from build123d import *

# Parameters (mm, degrees)
SKETCH_1_W          = 10
SKETCH_1_H          = 6
EXTRUDE_1_DEPTH     = 11.3
CUT_EXTRUDE_1_REACH = 18.239
SKETCH_3_W          = 3.4
SKETCH_3_H          = 3.4
CUT_EXTRUDE_2_DEPTH = 8
SKETCH_4_R          = 0.5
CUT_EXTRUDE_3_DEPTH = 0.1


with BuildPart() as part:
    # 草图1 → 凸台-拉伸1 (new body)
    with BuildSketch(Plane(origin=(0, 0, 0), x_dir=(1, 0, 0), z_dir=(0, 1, 0))):
        with Locations((5, 3)):
            Rectangle(SKETCH_1_W, SKETCH_1_H)
    extrude(amount=EXTRUDE_1_DEPTH)

    # 草图2 → 切除-拉伸1 (cut, up to next)
    with BuildSketch(Plane(origin=(0, 0, -6), x_dir=(-1, 0, 0), z_dir=(0, 0, -1)), mode=Mode.PRIVATE) as cut_extrude_1_sk1:
        Polygon((-10, 3.8), (-5.669872981, 11.3), (-10, 11.3), align=None)
    cut_extrude_1_tool1 = extrude(cut_extrude_1_sk1.sketch, amount=-CUT_EXTRUDE_1_REACH, mode=Mode.PRIVATE) & part.part
    add(cut_extrude_1_tool1.solids().sort_by_distance((8.556624, 8.8, -6))[0], mode=Mode.SUBTRACT)

    # 草图3 → 切除-拉伸2 (cut)
    with BuildSketch(Plane(origin=(9.145448267, 5.280127019, 0), x_dir=(0, 0, -1), z_dir=(0.8660254037844417, 0.4999999999999948, 0))):
        with Locations((3, 2.621023553)):
            Rectangle(SKETCH_3_W, SKETCH_3_H)
    extrude(amount=-CUT_EXTRUDE_2_DEPTH, mode=Mode.SUBTRACT)

    # 草图4 → 切除-拉伸3 (cut)
    with BuildSketch(Plane.XZ):
        with Locations(Location((5, -3, 0), (0, 0, 270))):
            Circle(SKETCH_4_R)
    extrude(amount=-CUT_EXTRUDE_3_DEPTH, mode=Mode.SUBTRACT)


solid = part.part
Geometry check sheet. Reference: the model listing, model coordinates, mm. A direction names the side the tool comes from. Coordinates: 2 decimals unless noted, no trailing zeros. Order: outer loops, then holes, each group sorted by start corner. A loop starts at its lowest first (then second) coordinate and runs counter-clockwise, first axis right, second up. Notation, with made-up numbers: (85, -39.5) - (118, -39.5) arc R29 ccw to (118, -17.5) - close; hole circle Ø1 at (70, 74). An arc over 180 degrees is marked (long way). One line per item, written item: value.
(1) Thickness scan on probe 1 along X at (y, z) = (0.05, -3); probe 2 along Z at (x, y) = (3.75, 3.75); probe 3 along Y at (x, z) = (6, -2.7). Record the ranges inside material, lowest first. Write a range as from..to.
Data:
probe 1: x = 0..4.5, 5.5..10
probe 2: z = -6..-4.7, -1.3..0
probe 3: y = 0..4.53, 8.45..10.73
(2) Release check for a two-part mould opening along Z. For faces 1 (the face through (4, 6, -6)), 2 (the face through (5.269, 4.106, -2.976)), 3 (the face through (4, 6, 0)), 4 (the face through (3, 11.3, -3)) record: +Z half, -Z half, draft (parallel to the pull), parting line (faces both ways), or undercut.
Data:
face 1: -Z half
face 2: undercut
face 3: +Z half
face 4: draft
(3) Sectioned sample at D-D (y = 7.75). Enter the section's corners in (x, z).
Data:
outline: (0, -6) - (7.72, -6) - (7.72, -4.7) - (4.78, -4.7) - (4.78, -1.3) - (7.72, -1.3) - (7.72, 0) - (0, 0) - close
(4) Access from +Z, -Z, +X, -X, +Y, -Y to the whole of each face (thin tool, end or side, straight path). Record for faces 5 (the face through (8.83, 5.83, -3.04)), 6 (the face through (5, 0.1, -3)), 7 (the face through (0.895, 3.571, -2.976)).
Data:
face 5: +Z, -Z, +X, +Y
face 6: -Y
face 7: none
(5) Sectioned sample at A-A (z = -4.5). Enter the section's corners in (x, y), and give its area (3 significant figures).
Data:
outline: (0, 0) - (10, 0) - (10, 3.8) - (8.68, 6.08) - (1.76, 2.08) - (0.06, 5.02) - (6.98, 9.02) - (5.67, 11.3) - (0, 11.3) - close
area: 69.6 mm^2
(6) Sectioned sample at C-C (x = 8.5). Enter the section's corners in (y, z), and give its area (3 significant figures).
Data:
outline: (0, -6) - (6.4, -6) - (6.4, -4.7) - (5.97, -4.7) - (5.97, -1.3) - (6.4, -1.3) - (6.4, 0) - (0, 0) - close
area: 36.9 mm^2
(7) Sectioned sample at B-B (x = 1.5). Enter the section's corners in (y, z), and give its area (3 significant figures).
Data:
outline: (0, -6) - (11.3, -6) - (11.3, 0) - (0, 0) - close; hole (2.52, -4.7) - (5.86, -4.7) - (5.86, -1.3) - (2.52, -1.3) - close
area: 56.5 mm^2
